Part model, mm, in its own coordinate system. Round coordinates to 2 decimals unless told otherwise and drop trailing zeros. Loops run counter-clockwise (first coordinate to the right, second up) from the corner with the lowest first, then second, coordinate; pieces in that order, holes last.
(1) Cut at A-A on x = -20. List the corners of the cut face in (y, z), then the cut area to 3 significant figures.
(2) Flat gauge pins, fed straight in: pin 1 (2 mm diameter, centred on y = -10, z = 11, fed in from +X); pin 2 (6 mm diameter, centred on y = -12.5, z = 6.5, fed in from -X); pin 3 (1 mm diameter, centred on y = 33, z = 8, fed in from -X). Where does each tip first touch, or does it go through?
(3) Cut at C-C on z = 11. List the corners of the cut face in (x, y), then the cut area to 3 significant figures.
(4) Cut at B-B on y = -9. List the corners of the cut face in (x, z).
(5) Probe probe 1 along Z at (x, y) = (103, 48); probe 2 along X at (y, z) = (32.5, 3.25); probe 3 along X at (y, z) = (21, 5). List the from-to ranges inside material, lowest first.
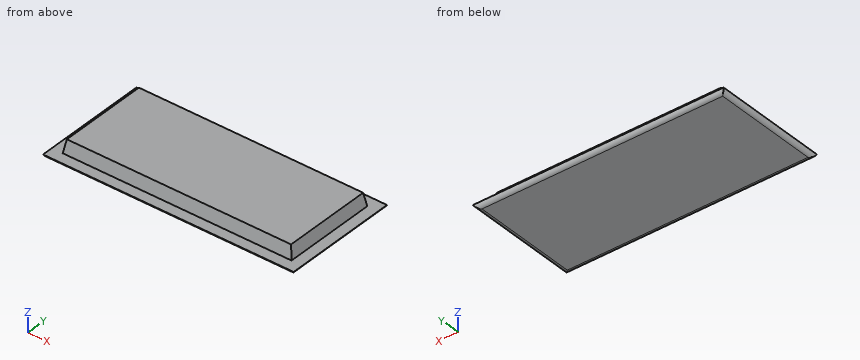
from build123d import *

# Parameters (mm, degrees)
F0_W         = 210
F0_H         = 86
F1_DEPTH     = 15
F0_W_2       = 230
F0_H_2       = 106
F2_DEPTH     = 3
F3_T1_DEPTH  = 252.9128784748
F3_T3_DEPTH  = 128.9128784748
F4_T4_DEPTH  = 272.3649311141
F4_T9_DEPTH  = 148.3649311141
F4_T14_DEPTH = 272.3649311141
F4_T19_DEPTH = 148.3649311141


# Not quite as in the source:
# - a fillet or chamfer that OpenCascade refuses, or shapes differently, is made with other operations: its cross-section is extruded or revolved along the edge and cut away or added


with BuildPart() as f1:
    # F0 (on Top) → F1 (new body)
    with BuildSketch(Plane.XY):
        Rectangle(F0_W, F0_H)
    extrude(amount=F1_DEPTH)

    # F0 (on Top) → F2 (join)
    with BuildSketch(Plane.XY):
        Rectangle(F0_W_2, F0_H_2)
        Rectangle(F0_W, F0_H, mode=Mode.SUBTRACT)
    extrude(amount=F2_DEPTH)

    # F3: fillet of radius 5 on 4 edges, made by hand

    # F3_s2 → F3_t1 (cut)
    with BuildSketch(Plane.YZ.offset(-126.4564392374)):
        with BuildLine():
            ThreePointArc((-53, 3), (-51.1560370926, 0.8166998673), (-48.417424305, 0))
            Line((-48.417424305, 0), (-53, 0))
            Line((-53, 0), (-53, 3))
        make_face()
        with BuildLine():
            ThreePointArc((53, 3), (51.1560370926, 0.8166998673), (48.417424305, 0))
            Line((48.417424305, 0), (53, 0))
            Line((53, 0), (53, 3))
        make_face()
    extrude(amount=F3_T1_DEPTH, mode=Mode.SUBTRACT)

    # F3_s4 → F3_t3 (cut)
    with BuildSketch(Plane.XZ.offset(-64.4564392374)):
        with BuildLine():
            ThreePointArc((115, 3), (113.1560370926, 0.8166998673), (110.417424305, 0))
            Line((110.417424305, 0), (115, 0))
            Line((115, 0), (115, 3))
        make_face()
        with BuildLine():
            ThreePointArc((-115, 3), (-113.1560370926, 0.8166998673), (-110.417424305, 0))
            Line((-110.417424305, 0), (-115, 0))
            Line((-115, 0), (-115, 3))
        make_face()
    extrude(amount=F3_T3_DEPTH, mode=Mode.SUBTRACT)

    # F4: chamfer of 12 x 2.1159237685 on 4 edges, made by hand


with BuildPart() as f4_tool2:
    # F4_s3 → F4_t4 (new body)
    with BuildSketch(Plane.YZ.offset(-136.1824655571)):
        Polygon((-43, 3), (-40.8840762315, 15), (-43, 15), align=None)
    extrude(amount=F4_T4_DEPTH)

    split(bisect_by=Plane.XY.offset(3), keep=Keep.TOP)


with BuildPart() as f1_1:
    add(f1.part)

    # F4_t1: cut F4_tool2
    add(f4_tool2.part, mode=Mode.SUBTRACT)


with BuildPart() as f4_tool7:
    # F4_s8 → F4_t9 (new body)
    with BuildSketch(Plane.XZ.offset(74.1824655571)):
        Polygon((105, 3), (102.8840762315, 15), (105, 15), align=None)
    extrude(amount=-F4_T9_DEPTH)

    split(bisect_by=Plane.XY.offset(3), keep=Keep.TOP)


with BuildPart() as f1_2:
    add(f1_1.part)

    # F4_t6: cut F4_tool7
    add(f4_tool7.part, mode=Mode.SUBTRACT)


with BuildPart() as f4_tool12:
    # F4_s13 → F4_t14 (new body)
    with BuildSketch(Plane.YZ.offset(136.1824655571)):
        Polygon((40.8840762315, 15), (43, 3), (43, 15), align=None)
    extrude(amount=-F4_T14_DEPTH)

    split(bisect_by=Plane.XY.offset(3), keep=Keep.TOP)


with BuildPart() as f1_3:
    add(f1_2.part)

    # F4_t11: cut F4_tool12
    add(f4_tool12.part, mode=Mode.SUBTRACT)


with BuildPart() as f4_tool17:
    # F4_s18 → F4_t19 (new body)
    with BuildSketch(Plane.XZ.offset(-74.1824655571)):
        Polygon((-102.8840762315, 15), (-105, 3), (-105, 15), align=None)
    extrude(amount=F4_T19_DEPTH)

    split(bisect_by=Plane.XY.offset(3), keep=Keep.TOP)


with BuildPart() as f1_4:
    add(f1_3.part)

    # F4_t16: cut F4_tool17
    add(f4_tool17.part, mode=Mode.SUBTRACT)


solid = f1_4.part
Final values:
1. outline: (-53, 3) arc R5 ccw to (-48.42, 0) - (48.42, 0) arc R5 ccw to (53, 3) - (43, 3) - (40.88, 15) - (-40.88, 15) - (-43, 3) - close
1. area: 1,320 mm2
2. pin 1: stops at x = 103.77
2. pin 2: stops at x = -104.91
2. pin 3: stops at x = -104.21
3. outline: (-103.59, -41.59) - (103.59, -41.59) - (103.59, 41.59) - (-103.59, 41.59) - close
3. area: 17,200 mm2
4. outline: (-115, 3) arc R5 ccw to (-110.42, 0) - (110.42, 0) arc R5 ccw to (115, 3) - (105, 3) - (102.88, 15) - (-102.88, 15) - (-105, 3) - close
5. probe 1: z = 0 to 3
5. probe 2: x = -104.96 to 104.96
5. probe 3: x = -104.65 to 104.65
